```python
from build123d import *

# Parameters (mm, degrees)
SKETCH2_R           = 4
SKETCH2_R_2         = 1.5
BOSS_EXTRUDE1_DEPTH = 1.5
SKETCH3_R           = 1.5
CUT_EXTRUDE1_DEPTH  = 1.5
SKETCH4_R           = 1.5
CUT_EXTRUDE2_DEPTH  = 1.5


with BuildPart() as part:
    # Sketch2 → Boss-Extrude1 (new body)
    with BuildSketch(Plane(origin=(0, 0, 0), x_dir=(1, 0, 0), z_dir=(0, 1, 0))):
        with BuildLine():
            Line((0, 0), (0, 9.381966011))
            ThreePointArc((0, 9.381966011), (0.5, 10.5), (0, 11.618033989))
            Line((0, 11.618033989), (0, 35.5))
            Line((0, 35.5), (15, 35.5))
            Line((15, 35.5), (23.677632731, 25.158400018))
            Line((23.677632731, 25.158400018), (129.929473623, 53.628494979))
            ThreePointArc((129.929473623, 53.628494979), (157.136079306, 48.289177788), (134.097880355, 32.863579259))
            Line((134.097880355, 32.863579259), (23.863280614, 3.331828071))
            Line((23.863280614, 3.331828071), (7.070663707, -8.426488874))
            Line((7.070663707, -8.426488874), (0, 0))
        make_face()
        with Locations(Location((142.429473623, 45.336933003, 0), (0, 0, 270))):
            Circle(SKETCH2_R, mode=Mode.SUBTRACT)
        with Locations(Location((8, 25.5, 0), (0, 0, 270))):
            Circle(SKETCH2_R_2, mode=Mode.SUBTRACT)
        with Locations(Location((14, 15.5, 0), (0, 0, 270))):
            Circle(SKETCH2_R_2, mode=Mode.SUBTRACT)
        with Locations(Location((8, 5.5, 0), (0, 0, 270))):
            Circle(SKETCH2_R_2, mode=Mode.SUBTRACT)
        with Locations(Location((142.429473623, 53.336933003, 0), (0, 0, 270))):
            Circle(SKETCH2_R_2, mode=Mode.SUBTRACT)
        with Locations(Location((151.929473623, 45.336933003, 0), (0, 0, 270))):
            Circle(SKETCH2_R_2, mode=Mode.SUBTRACT)
        with Locations(Location((142.429473623, 37.336933003, 0), (0, 0, 270))):
            Circle(SKETCH2_R_2, mode=Mode.SUBTRACT)
        with Locations(Location((132.929473623, 45.336933003, 0), (0, 0, 270))):
            Circle(SKETCH2_R_2, mode=Mode.SUBTRACT)
    extrude(amount=BOSS_EXTRUDE1_DEPTH)

    # Sketch3 → Cut-Extrude1 (cut)
    with BuildSketch(Plane(origin=(0, 1.5, 0), x_dir=(1, 0, 0), z_dir=(0, 1, 0))):
        with Locations((31.86, 6.64)):
            Circle(SKETCH3_R)
    extrude(amount=-CUT_EXTRUDE1_DEPTH, mode=Mode.SUBTRACT)

    # Sketch4 → Cut-Extrude2 (cut)
    with BuildSketch(Plane(origin=(0, 1.5, 0), x_dir=(1, 0, 0), z_dir=(0, 1, 0))):
        with Locations(Location((75.037341097, 27.279265517, 0), (0, 0, 270))):
            Circle(SKETCH4_R)
        with Locations(Location((104.015115886, 35.04383687, 0), (0, 0, 270))):
            Circle(SKETCH4_R)
    extrude(amount=-CUT_EXTRUDE2_DEPTH, mode=Mode.SUBTRACT)


solid = part.part
```
Work out the finished part from the listing and answer in its coordinate system (mm). A direction names the side the tool comes from. Coordinates: 2 decimals unless noted, no trailing zeros. Loops run counter-clockwise (first coordinate to the right, second up) from the corner with the lowest first, then second, coordinate; pieces in that order, holes last.
1) Consider probe 1 along Z at (x, y) = (142.5, 0.4); probe 2 along Z at (x, y) = (143.5, 0.8); probe 3 along Z at (x, y) = (11.5, 0.75). Determine where each line is inside the solid, lowest interval first.
Results:
probe 1: z = -60.34 to -54.84, -51.84 to -49.34, -41.34 to -38.84, -35.84 to -30.34
probe 2: z = -60.3 to -54.39, -52.29 to -49.19, -41.48 to -38.39, -36.29 to -30.38
probe 3: z = -35.5 to 5.33
2) Section C-C (x = 65) is taken. Give the vertices of the cut face in (y, z), plus the area to 3 significant figures.
Results:
outline: (0, -36.23) - (1.5, -36.23) - (1.5, -14.35) - (0, -14.35) - close
area: 32.8 mm2
3) Section B-B (z = -15.5) is taken. Give the vertices of the cut face in (x, y), plus the area to 3 significant figures.
Results:
outline: (0, 0) - (12.5, 0) - (12.5, 1.5) - (0, 1.5) - close; (15.5, 0) - (69.28, 0) - (69.28, 1.5) - (15.5, 1.5) - close
area: 99.4 mm2
4) For faces 5 (the flat face through (76.06, 0.74, -39.194)), 6 (the cylindrical face through (132.995, 0.74, -46.835)), determine the directions among +Z, -Z, +X, -X, +Y, -Y from which every point of the face is accessible in a straight line to the end or side of a thin tool.
Results:
face 5: -Z, +Y, -Y
face 6: +Y, -Y
5) Section A-A (y = 0.8) is taken. Give the number of separate pieces and of enclosed holes in the cut face, plus the area to 3 significant figures.
Results:
separate pieces: 1
enclosed holes: 10
area: 3,760 mm2
6) Section D-D (x = 11) is taken. Give the vertices of the cut face in (y, z).
Results:
outline: (0, -35.5) - (1.5, -35.5) - (1.5, 5.68) - (0, 5.68) - close
7) A flat-ended cylindrical pin translates along its axis: pin 1 (10 mm diameter, centred on x = 42, z = -19.5, fed in from -Y). Find the tip coordinate at first contact, or state that the pin passes through.
Results:
pin 1: stops at y = 0
8) For a pull along Z with two mould halves and no side action, classify faces 1 (the cylindrical face through (145.802, 0.74, -43.187)), 2 (the cylindrical face through (14, 1, -17)), 3 (the flat face through (80, 1.5, -26)), 4 (the flat face through (84.31, 0.74, -19.525)) as +Z half, -Z half, draft (parallel to the pull), parting line (faces both ways), or undercut.
Results:
face 1: undercut
face 2: undercut
face 3: draft
face 4: +Z half
